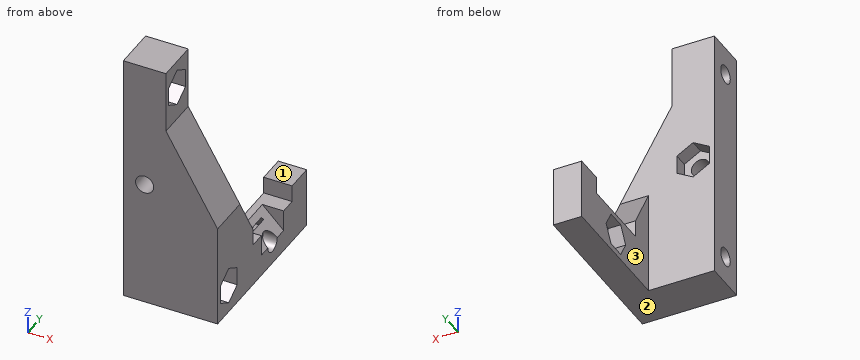
from build123d import *

# Parameters (mm, degrees)
SALIENTE_EXTRUIR1_DEPTH = 7.6
CORTAR_EXTRUIR1_REACH   = 18.6
CROQUIS2_R              = 1.6
CROQUIS3_W              = 5
CROQUIS3_H              = 4.9
SALIENTE_EXTRUIR2_DEPTH = 3
SALIENTE_EXTRUIR3_DEPTH = 5
SALIENTE_EXTRUIR4_DEPTH = 7.621024
SALIENTE_EXTRUIR5_DEPTH = 7.5
CROQUIS7_W              = 7.5
CROQUIS7_H              = 7.5
SALIENTE_EXTRUIR6_DEPTH = 26.778976
CORTAR_EXTRUIR2_REACH   = 18.6
CROQUIS8_R              = 1.6
CORTAR_EXTRUIR3_DEPTH   = 2.5
CORTAR_EXTRUIR4_DEPTH   = 2.5
CORTAR_EXTRUIR5_DEPTH   = 12.1
CORTAR_EXTRUIR6_REACH   = 9.5
CROQUIS12_R             = 1.6
CORTAR_EXTRUIR7_DEPTH   = 2.5
CORTAR_EXTRUIR8_DEPTH   = 3.75


with BuildPart() as part:
    # Croquis1 → Saliente-Extruir1 (new body)
    with BuildSketch(Plane.XY):
        Polygon((0, 0), (16.6, 0), (16.6, 30), (11.6, 30), (11.6, 7.5), (0, 7.5), align=None)
    extrude(amount=SALIENTE_EXTRUIR1_DEPTH)

    # Croquis2 → Cortar-Extruir1 (cut, up to next)
    with BuildSketch(Plane(origin=(16.6, 0, 0), x_dir=(0, 0, -1), z_dir=(1, 0, 0)), mode=Mode.PRIVATE) as cortar_extruir1_sk1:
        with Locations((-3.85, 18.5)):
            Circle(CROQUIS2_R)
    cortar_extruir1_tool1 = extrude(cortar_extruir1_sk1.sketch, amount=-CORTAR_EXTRUIR1_REACH, mode=Mode.PRIVATE) & part.part
    add(cortar_extruir1_tool1.solids().sort_by_distance((16.6, 18.5, 3.85))[0], mode=Mode.SUBTRACT)

    # Croquis3 → Saliente-Extruir2 (add)
    with BuildSketch(Plane.XY.offset(7.6)):
        with Locations((14.1, 27.55)):
            Rectangle(CROQUIS3_W, CROQUIS3_H)
        Polygon((11.6, 11.9), (16.6, 11.9), (16.6, 0), (0, 0), (0, 7.5), (11.6, 7.5), align=None)
    extrude(amount=SALIENTE_EXTRUIR2_DEPTH)

    # Croquis4 → Saliente-Extruir3 (add)
    with BuildSketch(Plane(origin=(16.6, 0, 0), x_dir=(0, 0, -1), z_dir=(1, 0, 0))):
        Polygon((-10.6, 7.5), (-18.221023553, 7.5), (-10.6, 11.9), align=None)
    extrude(amount=-SALIENTE_EXTRUIR3_DEPTH)

    # Croquis5 → Saliente-Extruir4 (add)
    with BuildSketch(Plane.XY.offset(10.6)):
        Polygon((16.6, 0), (16.6, 7.5), (11.6, 7.5), (0, 7.5), (0, 0), align=None)
    extrude(amount=SALIENTE_EXTRUIR4_DEPTH)

    # Croquis6 → Saliente-Extruir5 (add)
    with BuildSketch(Plane.XZ):
        Polygon((7.5, 18.221023553), (7.5, 33.982685902), (16.6, 18.221023553), align=None)
    extrude(amount=-SALIENTE_EXTRUIR5_DEPTH)

    # Croquis7 → Saliente-Extruir6 (add)
    with BuildSketch(Plane.XY.offset(18.221023553)):
        with Locations((3.75, 3.75)):
            Rectangle(CROQUIS7_W, CROQUIS7_H)
    extrude(amount=SALIENTE_EXTRUIR6_DEPTH)

    # Croquis8 → Cortar-Extruir2 (cut, up to next)
    with BuildSketch(Plane.ZY, mode=Mode.PRIVATE) as cortar_extruir2_sk1:
        with Locations((40, 3.75)):
            Circle(CROQUIS8_R)
    cortar_extruir2_tool1 = extrude(cortar_extruir2_sk1.sketch, amount=-CORTAR_EXTRUIR2_REACH, mode=Mode.PRIVATE) & part.part
    add(cortar_extruir2_tool1.solids().sort_by_distance((0, 3.75, 40))[0], mode=Mode.SUBTRACT)
    # Croquis8 → Cortar-Extruir2 (cut, up to next)
    with BuildSketch(Plane.ZY, mode=Mode.PRIVATE) as cortar_extruir2_sk2:
        with Locations((5, 3.75)):
            Circle(CROQUIS8_R)
    cortar_extruir2_tool2 = extrude(cortar_extruir2_sk2.sketch, amount=-CORTAR_EXTRUIR2_REACH, mode=Mode.PRIVATE) & part.part
    add(cortar_extruir2_tool2.solids().sort_by_distance((0, 3.75, 5))[0], mode=Mode.SUBTRACT)

    # Croquis9 → Cortar-Extruir3 (cut)
    with BuildSketch(Plane.ZY.offset(-11.6)):
        Polygon((1, 16.854551733), (3.85, 15.209103466), (6.7, 16.854551733), (6.7, 20.145448267), (3.85, 21.790896534), (1, 20.145448267), align=None)
    extrude(amount=-CORTAR_EXTRUIR3_DEPTH, mode=Mode.SUBTRACT)

    # Croquis10 → Cortar-Extruir4 (cut)
    with BuildSketch(Plane(origin=(7.5, 0, 0), x_dir=(0, 0, -1), z_dir=(1, 0, 0))):
        Polygon((-38.354551733, 6.6), (-41.645448267, 6.6), (-43.290896534, 3.75), (-41.645448267, 0.9), (-38.354551733, 0.9), (-36.709103466, 3.75), align=None)
    extrude(amount=-CORTAR_EXTRUIR4_DEPTH, mode=Mode.SUBTRACT)

    # Croquis11 → Cortar-Extruir5 (cut)
    with BuildSketch(Plane(origin=(16.6, 0, 0), x_dir=(0, 0, -1), z_dir=(1, 0, 0))):
        Polygon((-6.645448267, 0.9), (-3.354551733, 0.9), (-1.709103466, 3.75), (-3.354551733, 6.6), (-6.645448267, 6.6), (-8.290896534, 3.75), align=None)
    extrude(amount=-CORTAR_EXTRUIR5_DEPTH, mode=Mode.SUBTRACT)

    # Croquis12 → Cortar-Extruir6 (cut, up to next)
    with BuildSketch(Plane(origin=(0, 7.5, 0), x_dir=(1, 0, 0), z_dir=(0, 1, 0)), mode=Mode.PRIVATE) as cortar_extruir6_sk1:
        with Locations((3.75, -22.5)):
            Circle(CROQUIS12_R)
    cortar_extruir6_tool1 = extrude(cortar_extruir6_sk1.sketch, amount=-CORTAR_EXTRUIR6_REACH, mode=Mode.PRIVATE) & part.part
    add(cortar_extruir6_tool1.solids().sort_by_distance((3.75, 7.5, 22.5))[0], mode=Mode.SUBTRACT)

    # Croquis13 → Cortar-Extruir7 (cut)
    with BuildSketch(Plane.XZ.offset(-7.5)):
        Polygon((6.6, 20.854551733), (6.6, 24.145448267), (3.75, 25.790896534), (0.9, 24.145448267), (0.9, 20.854551733), (3.75, 19.209103466), align=None)
    extrude(amount=CORTAR_EXTRUIR7_DEPTH, mode=Mode.SUBTRACT)

    # Croquis14 → Cortar-Extruir8 (cut, symmetric)
    with BuildSketch(Plane(origin=(0, 18.5, 0), x_dir=(-1, 0, 0), z_dir=(0, 1, 0))):
        Polygon((-16.6, 7.6), (-16.6, 3.85), (-12.85, 7.6), align=None)
    extrude(amount=CORTAR_EXTRUIR8_DEPTH, both=True, mode=Mode.SUBTRACT)


solid = part.part
The model under review builds one solid part; all positions refer to its coordinate system, in mm. Face numbers are marked on the shaded views. A direction names the side the tool comes from. Round coordinates to 2 decimals unless told otherwise and drop trailing zeros. Order: outer loops, then holes, each group sorted by start corner. A loop starts at its lowest first (then second) coordinate and runs counter-clockwise, first axis right, second up. Notation, with made-up numbers: (66, 75) -> (111, 75) arc R33 cw to (111, 108) -> close; hole circle Ø1 at (44.5, -17.5). An arc over 180 degrees is marked (long way). Return JSON: item names as keys, results as strings.
1. Take a section at B-B (z = 40). Write out the cut boundary in (x, y).
Answer block:
{"outline": "(0, 0) -> (7.5, 0) -> (7.5, 0.9) -> (5, 0.9) -> (5, 2.15) -> (0, 2.15) -> close; (0, 5.35) -> (5, 5.35) -> (5, 6.6) -> (7.5, 6.6) -> (7.5, 7.5) -> (0, 7.5) -> close"}
2. Take a section at C-C (x = 12.25). Write out the cut boundary in (y, z), then the cut area to 3 significant figures.
Answer block:
{"outline": "(0, 0) -> (30, 0) -> (30, 10.6) -> (25.1, 10.6) -> (25.1, 7.6) -> (11.9, 7.6) -> (11.9, 10.6) -> (7.5, 18.22) -> (7.5, 25.76) -> (0, 25.76) -> close; hole (0.9, 3.35) -> (3.75, 1.71) -> (6.6, 3.35) -> (6.6, 6.65) -> (3.75, 8.29) -> (0.9, 6.65) -> close; hole (15.21, 3.85) -> (16.85, 1) -> (20.15, 1) -> (21.79, 3.85) -> (20.15, 6.7) -> (16.85, 6.7) -> close", "area": "353 mm²"}
3. For L1, parallel to Y at x = 16, z = 3.85; L2, parallel to Y at x = 2.1, z = 40; L3, parallel to Z at x = 3.75, y = 2.45, list the stretches that pass through material, from the lowest coordinate up. Write a range as [from, to].
Answer block:
{"L1": "y = [0, 0.9], [6.6, 16.9], [20.1, 30]", "L2": "y = [0, 2.15], [5.35, 7.5]", "L3": "z = [0, 4.07], [5.93, 20.9], [24.1, 39.07], [40.93, 45]"}
4. Take a section at D-D (z = 22.5). Write out the cut boundary in (x, y), then the cut area to 3 significant figures.
Answer block:
{"outline": "(0, 0) -> (2.15, 0) -> (2.15, 5) -> (0.9, 5) -> (0.9, 7.5) -> (0, 7.5) -> close; (5.35, 0) -> (14.13, 0) -> (14.13, 7.5) -> (6.6, 7.5) -> (6.6, 5) -> (5.35, 5) -> close", "area": "75.7 mm²"}
5. Insertion check: P1, Ø12, axis at y = 17, z = 8, coming from the -X side; P2, Ø1.1, axis at x = 15.5, z = 6, coming from the -Y side; P3, Ø2.5, axis at y = 17.5, z = 3.5, coming from the -X side; P4, Ø0.8, axis at x = 12.5, y = 19, coming from the +Z side. Each pin has a flat end and moves straight along its axis. Give the tip position at first contact, or say it passes through.
Answer block:
{"P1": "stops at x = 11.6", "P2": "stops at y = 0", "P3": "stops at x = 14.1", "P4": "stops at z = 7.6"}
6. Take a section at A-A (y = 18.5). Write out the cut boundary in (x, z).
Answer block:
{"outline": "(11.6, 0) -> (16.6, 0) -> (16.6, 2.25) -> (14.1, 2.25) -> (14.1, 1) -> (11.6, 1) -> close; (11.6, 6.7) -> (13.75, 6.7) -> (12.85, 7.6) -> (11.6, 7.6) -> close; (14.1, 5.45) -> (15, 5.45) -> (14.1, 6.35) -> close"}
7. For the marked faces 1, 2 and 3, list the 3-axis set-ups (+Z, -Z, +X, -X, +Y, -Y) from which the entire face can be reached by the end or side of a thin tool; tool diameter is ignored.
Answer block:
{"face 1": "+Z, +X, -X, +Y", "face 2": "-Z, +X, -X, +Y, -Y", "face 3": "+Z, -Z, -X, +Y"}
